CAD build for the part. Positions are in the model's coordinates, mm. Coordinates: 2 decimals unless noted, no trailing zeros. Loops run counter-clockwise (first coordinate to the right, second up) from the corner with the lowest first, then second, coordinate; pieces in that order, holes last. Notation, with made-up numbers: (-18, 61) -> (0, 61) arc R20 cw to (0, 82) -> close; hole circle Ø7 at (-33.75, -14). An arc over 180 degrees is marked (long way). Answer as a JSON object with one key per item and string values. Group by question number.
from build123d import *

# Parameters (mm, degrees)
F2_R     = 1.9
F3_DEPTH = 1.6
F5_START = -1.601
F5_DEPTH = 9.002


with BuildPart() as f1:
    # F0 (on Front) → F1 (revolve)
    with BuildSketch(Plane.XZ):
        Polygon((-1.6, 14.6), (-1.6, 2.8), (7.4, 2.8), (7.4, 4), (0, 4), (0, 14.6), align=None)
    revolve(axis=Axis((3.7, 0, 0), (1, 0, 0)))

    # F2 (on Right) → F3 (cut, through all)
    with BuildSketch(Plane.YZ):
        with Locations((0, 11.6)):
            Circle(F2_R)
        with Locations((-10.0458946839, 5.8)):
            Circle(F2_R)
        with Locations((-10.0458946839, -5.8)):
            Circle(F2_R)
        with Locations((0, -11.6)):
            Circle(F2_R)
        with Locations((10.0458946839, -5.8)):
            Circle(F2_R)
        with Locations((10.0458946839, 5.8)):
            Circle(F2_R)
    extrude(amount=-F3_DEPTH, mode=Mode.SUBTRACT)

    # F4 (on Right) → F5 (intersect)
    with BuildSketch(Plane.YZ.offset(F5_START)):
        with BuildLine():
            ThreePointArc((8.5458946839, 8.3980762114), (4.8486315613, 8.3980762114), (3, 11.6))
            ThreePointArc((3, 11.6), (0, 14.6), (-3, 11.6))
            ThreePointArc((-3, 11.6), (-4.8486315613, 8.3980762114), (-8.5458946839, 8.3980762114))
            ThreePointArc((-8.5458946839, 8.3980762114), (-12.6439708953, 7.3), (-11.5458946839, 3.2019237886))
            ThreePointArc((-11.5458946839, 3.2019237886), (-9.6972631226, 0), (-11.5458946839, -3.2019237886))
            ThreePointArc((-11.5458946839, -3.2019237886), (-12.6439708953, -7.3), (-8.5458946839, -8.3980762114))
            ThreePointArc((-8.5458946839, -8.3980762114), (-4.8486315613, -8.3980762114), (-3, -11.6))
            ThreePointArc((-3, -11.6), (0, -14.6), (3, -11.6))
            ThreePointArc((3, -11.6), (4.8486315613, -8.3980762114), (8.5458946839, -8.3980762114))
            ThreePointArc((8.5458946839, -8.3980762114), (12.6439708953, -7.3), (11.5458946839, -3.2019237886))
            ThreePointArc((11.5458946839, -3.2019237886), (9.6972631226, 0), (11.5458946839, 3.2019237886))
            ThreePointArc((11.5458946839, 3.2019237886), (12.6439708953, 7.3), (8.5458946839, 8.3980762114))
        make_face()
    extrude(amount=F5_DEPTH, mode=Mode.INTERSECT)


solid = f1.part
Item 1: Band-saw the part on D-D, the plane x = 2.5. List the corners of the cut face in (y, z).
Item 2: Band-saw the part on A-A, the plane z = 5.8. List the corners of the cut face in (x, y).
Item 3: Drill centre lines: L1, parallel to Z at x = -0.4, y = 0; L2, parallel to Z at x = 6, y = 0. Where is each one in solid material? Low to high.
Item 4: Band-saw the part on B-B, the plane z = 0. List the corners of the cut face in (x, y).
Item 5: Flat gauge pins, fed straight in: P1, Ø5, axis at x = 5.5, z = -5.5, coming from the +Y side; P2, Ø4, axis at x = 5, z = 3, coming from the +Y side; P3, Ø3.5, axis at y = 0, z = 0, coming from the -X side; P4, Ø5, axis at y = 0, z = -11.6, coming from the +X side. Where does each tip first touch, or does it go through?
Item 6: Band-saw the part on C-C, the plane y = 2.25. List the corners of the cut face in (x, z), and give its area (3 significant figures).
Item 7: Pull direction Y, two halves, no side cores. Call faces 1 (the cylindrical face through (-0.811, 4.802, -8.426)), 2 (the cylindrical face through (-0.8, -9.7, 0.1)), 3 (the cylindrical face through (3.648, 3.905, -0.867)), 4 (the flat face through (0, -3, -3)): +Y half, -Y half, draft (parallel to the pull), parting line (faces both ways), or undercut.
Reply:
{
 "1": {"outline": "circle Ø8 at (0, 0); hole circle Ø5.6 at (0, 0)"},
 "2": {"outline": "(-1.6, -13.05) -> (0, -13.05) -> (0, -11.95) -> (-1.6, -11.95) -> close; (-1.6, -8.15) -> (0, -8.15) -> (0, 8.15) -> (-1.6, 8.15) -> close; (-1.6, 11.95) -> (0, 11.95) -> (0, 13.05) -> (-1.6, 13.05) -> close"},
 "3": {"L1": "-14.6 to -13.5, -9.7 to -2.8, 2.8 to 9.7, 13.5 to 14.6", "L2": "-4 to -2.8, 2.8 to 4"},
 "4": {"outline": "(-1.6, -9.7) -> (0, -9.7) -> (0, -4) -> (7.4, -4) -> (7.4, -2.8) -> (-1.6, -2.8) -> close; (-1.6, 2.8) -> (7.4, 2.8) -> (7.4, 4) -> (0, 4) -> (0, 9.7) -> (-1.6, 9.7) -> close"},
 "5": {"P1": "y = 2.65", "P2": "y = 3.87", "P3": "through", "P4": "x = 0"},
 "6": {"outline": "(-1.6, -13.58) -> (0, -13.58) -> (0, -3.31) -> (7.4, -3.31) -> (7.4, -1.67) -> (-1.6, -1.67) -> close; (-1.6, 1.67) -> (7.4, 1.67) -> (7.4, 3.31) -> (0, 3.31) -> (0, 13.58) -> (-1.6, 13.58) -> close", "area": "62.4 mm²"},
 "7": {"face 1": "undercut", "face 2": "-Y half", "face 3": "parting line", "face 4": "draft"}
}
